Could you check a few things on this model? Use its own coordinates, in mm. Coordinates: 2 decimals unless noted, no trailing zeros. Order: outer loops, then holes, each group sorted by start corner. A loop starts at its lowest first (then second) coordinate and runs counter-clockwise, first axis right, second up. Notation, with made-up numbers: (-9.5, 65.25) -> (14.5, 65.25) arc R15 ccw to (14.5, 93.25) -> close; hole circle Ø7 at (55, 4). An arc over 180 degrees is marked (long way). Put each result on its own line as item: value. Start each with the question number.
Q1. Please list where these lines run through material, in increasing order: line 1 along Z through (x, y) = (-123.45, 4); line 2 along X through (y, z) = (9, 9.25); line 3 along Z through (x, y) = (-55.5, 2).
Q2. If we section it at B-B (y = 3.5): Count the separate pieces of the cut face and the enclosed holes in it, and give its area (3 significant figures).
Q3. Will this pin go through, and if not, where does the flat tip stop? pin 1 (3.5 mm diameter, centred on x = -46.55, z = 5, fed in from +Y).
Q4. If we section it at A-A (x = -6.1): Please give me the cut outline in (y, z), and give its area (3 significant figures).
Q5. If we section it at D-D (x = -123.45): Please give me the cut outline in (y, z).
Autodesk Inventor part; units mm, degrees
ref_plane "YZ Plane" through (0, 0, 0) normal (1, 0, 0) x (0, 1, 0)
ref_plane "XZ Plane" through (0, 0, 0) normal (0, 1, 0) x (-1, 0, 0)
ref_plane "XY Plane" through (0, 0, 0) normal (0, 0, 1) x (1, 0, 0)
sketch "Sketch1" plane through (0, 0, 0) normal (0, 1, 0) x (-1, 0, 0)
  line L0 (0, 0) -> (170, 0)
  line L1 (170, 0) -> (170, 10)
  line L2 (170, 10) -> (0, 10)
  line L3 (0, 10) -> (0, 0)
  dimension "d0" = 170
  dimension "d1" = 10
extrude "Extrusion1" add sketch "Sketch1" along normal blind 10
sketch "Sketch2" plane through (0, 10, 0) normal (0, 1, 0) x (1, 0, 0)
  line L0 (0, -10) -> (0, 0)
  line L1 (0, -5) -> (-2.2, -5)
  circle A0 centre (-6.1, -5) radius 3.9
  line L2 (0, 0) -> (-170, 0)
  line L3 (-170, -10) -> (0, -10)
  circle A1 centre (-75, -5) radius 1.5
  circle A2 centre (-95, -5) radius 1.5
  dimension "d4" = 2.2
  dimension "d8" = 3
  dimension "d9" = 3
extrude "Extrusion2" cut sketch "Sketch2" against normal blind 10 contours A1
extrude "Extrusion3" cut sketch "Sketch2" against normal blind 10 contours A2
extrude "Extrusion4" cut sketch "Sketch2" against normal blind 10 contours A0
sketch "Sketch3" plane through (0, 10, 0) normal (0, 1, 0) x (1, 0, 0)
  line L0 (-170, 0) -> (-170, -10)
  line L1 (-170, -5) -> (-10, -5)
  circle A0 centre (-6.1, -5) radius 3.9
  line L2 (-165.7, -5) -> (-163.45, -5)
  circle A1 centre (-163.45, -5) radius 2.25
  circle A2 centre (-153.45, -5) radius 2.25
  circle A3 centre (-143.45, -5) radius 2.25
  circle A4 centre (-133.45, -5) radius 2.25
  circle A5 centre (-123.45, -5) radius 2.25
  circle A6 centre (-113.45, -5) radius 2.25
  circle A7 centre (-103.45, -5) radius 2.25
  circle A8 centre (-95, -5) radius 1.5
  line L3 (-93.5, -5) -> (-93.5, -7.9104)
  circle A9 centre (-75, -5) radius 1.5
  line L4 (-76.5, -5) -> (-76.5, -7.25)
  line L5 (-93.5, -5) -> (-76.5, -5)
  line L6 (-85, -5) -> (-93.5, -5)
  line L7 (-85, -5) -> (-76.5, -5)
  circle A10 centre (-80.75, -5) radius 2.25
  circle A11 centre (-89.25, -5) radius 2.25
  line L8 (-10, -5) -> (-12, -5)
  line L9 (-10, -5) -> (-14.3, -5)
  line L10 (-14.3, -5) -> (-16.55, -5)
  circle A12 centre (-16.55, -5) radius 2.25
  circle A13 centre (-26.55, -5) radius 2.25
  circle A14 centre (-36.55, -5) radius 2.25
  circle A15 centre (-46.55, -5) radius 2.25
  circle A16 centre (-56.55, -5) radius 2.25
  circle A17 centre (-66.55, -5) radius 2.25
  point P0 (0, 0)
  point P1 (-155.7, -5)
  point P2 (-145.7, -5)
  point P3 (-135.7, -5)
  point P4 (-125.7, -5)
  point P5 (-115.7, -5)
  point P6 (-105.7, -5)
  point P7 (-24.3, -5)
  point P8 (-34.3, -5)
  point P9 (-44.3, -5)
  point P10 (-54.3, -5)
  point P11 (-64.3, -5)
  dimension "d20" = 10
  dimension "d32" = 10
extrude "Extrusion5" cut sketch "Sketch3" against normal blind 10 contours A1 L1 | L1 A1 | L1 A12 | L1 A12 | A2 L1 | L1 A2 | A3 L1 | L1 A3 | A4 L1 | L1 A4 | A5 L1 | L1 A5 | A6 L1 | L1 A6 | A7 L1 | L1 A7 | A11 L1 | L1 A11 | A10 L1 | L1 A10 | A17 L1 | L1 A17 | A16 L1 | L1 A16 | A15 L1 | L1 A15 | A14 L1 | L1 A14 | A13 L1 | L1 A13
thread "Thread1"
thread "Thread2"
sketch "Sketch4" plane through (0, 10, 0) normal (0, 1, 0) x (1, 0, 0)
  circle A0 centre (-16.55, -5) radius 2.25
  circle A1 centre (-16.55, -5) radius 2.25
  point P0 (0, 0)
extrude "Extrusion6" add sketch "Sketch4" against normal blind 10
sketch "Sketch5" plane through (0, 0, 10) normal (1, 0, 0) x (0, 0, -1)
  line L0 (10, 0) -> (0, 0)
  line L1 (0, 0) -> (0, 10)
  line L2 (10, 0) -> (0, 0)
  line L3 (0, 0) -> (0, 10)
  line L4 (0, 10) -> (10, 10)
  line L5 (10, 10) -> (10, 0)
extrude "Extrusion7" add sketch "Sketch5" along normal blind 10
sketch "Sketch6" plane through (10, 0, 10) normal (1, 0, 0) x (0, 0, -1)
  line L0 (0, 0) -> (10, 0)
  line L1 (0, 10) -> (0, 0)
  line L2 (10, 0) -> (0, 0)
  line L3 (0, 0) -> (0, 10)
  line L4 (0, 10) -> (10, 10)
  line L5 (10, 10) -> (10, 0)
extrude "Extrusion8" add sketch "Sketch6" along normal blind 10
sketch "Sketch7" plane through (0, 10, 0) normal (0, 1, 0) x (1, 0, 0)
  point P0 (0, 0)
fillet "Fillet3" radius 1 11 edges at (-75, 10, 10) (-75, 0, 10) (-75, 10, 0) (20, 5, 10) (20, 5, 0) (20, 0, 5) (-170, 10, 5) (-170, 5, 10) (-170, 5, 0) (-170, 0, 5) (-75, 0, 0)
fillet "Fillet4" radius 1 3 edges at (19.7071, 9.7071, 9.7071) (19.7071, 9.7071, 0.2929) (20, 10, 5)
sketch "Sketch8" plane through (19, 1, 0) normal (0, 0, -1) x (-1, 0, 0)
  point P0 (19, -1)
sketch "Sketch9" plane through (0, 10, 0) normal (0, 1, 0) x (1, 0, 0)
  circle A0 centre (-6.1, -5) radius 3.9
  circle A1 centre (-6.1, -5) radius 2.5
  point P0 (0, 0)
  dimension "d53" = 5
extrude "Extrusion9" add sketch "Sketch9" against normal blind 10
properties part number "brazo apoyo"
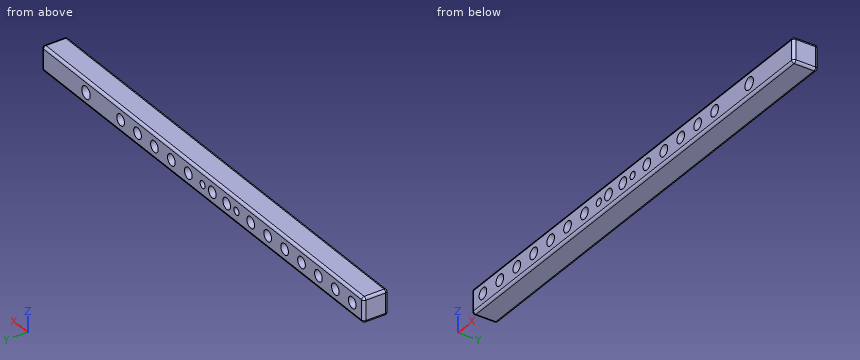
The answers:
1. line 1: 0 to 2.75, 7.25 to 10
1. line 2: -169.97 to 19.97
1. line 3: 0 to 3.01, 6.99 to 10
2. separate pieces: 1
2. enclosed holes: 17
2. area: 1,640 mm^2
3. pin 1: through
4. outline: (0, 1) arc R1 ccw to (1, 0) -> (9, 0) arc R1 ccw to (10, 1) -> (10, 2.5) -> (0, 2.5) -> close; (0, 7.5) -> (10, 7.5) -> (10, 9) arc R1 ccw to (9, 10) -> (1, 10) arc R1 ccw to (0, 9) -> close
4. area: 49.1 mm^2
5. outline: (0, 1) arc R1 ccw to (1, 0) -> (9, 0) arc R1 ccw to (10, 1) -> (10, 2.75) -> (0, 2.75) -> close; (0, 7.25) -> (10, 7.25) -> (10, 9) arc R1 ccw to (9, 10) -> (1, 10) arc R1 ccw to (0, 9) -> close
